Source: CAD feature listing. Evaluate the final solid. Frame: model axes, mm. A direction names the side the tool comes from. Give positions to 0.01 mm unless a question says otherwise; leave off trailing zeros. Order: outer loops, then holes, each group sorted by start corner. A loop starts at its lowest first (then second) coordinate and runs counter-clockwise, first axis right, second up.
from build123d import *

# Parameters (mm, degrees)
F0_R     = 15.875
F0_R_2   = 9.525
F1_DEPTH = 127
F2_R     = 9.525
F3_DEPTH = 12.7
F5_SCALE = 0.5


with BuildPart() as f1:
    # F0 (on Right) → F1 (new body)
    with BuildSketch(Plane.YZ):
        Circle(F0_R)
        Circle(F0_R_2, mode=Mode.SUBTRACT)
    extrude(amount=F1_DEPTH)

    # F2 (on face) → F3 (join)
    with BuildSketch(Plane.YZ.offset(127)):
        Polygon((-0.4526267682, -15.8685460584), (13.5162506236, -8.3262593089), (13.9688773918, 7.5422867496), (0.4526267682, 15.8685460584), (-13.5162506236, 8.3262593089), (-13.9688773918, -7.5422867496), align=None)
        Circle(F2_R, mode=Mode.SUBTRACT)
    extrude(amount=F3_DEPTH)

    # F4: F1 across face


with BuildPart() as f1_1:
    add(f1.part)
    add(f1.part.mirror(Plane.YZ.offset(139.7)))


with BuildPart() as f1_2:
    # F5: moved
    add(f1_1.part.scale(F5_SCALE))


solid = f1_2.part
(1) Section B-B, the plane x = 30. Return loops of the section in (y, z) (1 decimal), plus the area to 3 significant figures.
(2) Pin query (flat end, axial travel): pin 1 Ø3 at (x, z) = (62.5, 5) entering from -Y. Return the tip coordinate at first contact, or that it passes through.
(3) Line query: line 1 along Z through (x, y) = (35, 0); line 2 along Y through (x, z) = (109, -0.5); line 3 along Z through (x, y) = (77, -4). Output: solid intervals per line, ascending.
(4) Section C-C, the plane y = 1.5. Return loops of the section in (x, z).
(5) Access query for faces 4 (the flat face through (76.2, 4, 6)), 5 (the flat face through (63.5, -4, -6)), 6 (the flat face through (63.5, 4, -6)). Directions: +Z, -Z, +X, -X, +Y, -Y. A direction counts if a zero-diameter tool reaches every point of the face in a straight line with its end or side. Return the directions, or none.
(6) Draft query along X for faces 1 (the cylindrical face through (31.31, -1.72, -7.75)), 2 (the flat face through (69.939, -3.653, -5.824)), 3 (the flat face through (139.7, 0, -5)). Return one class per face: +X half, -X half, draft (parallel to the pull), parting line (faces both ways), or undercut.
(7) Section A-A, the plane z = 0. Return loops of the section in (x, y).
Checks:
1. outline: circle Ø15.9 at (0, 0); hole circle Ø9.5 at (0, 0)
1. area: 127 mm2
2. pin 1: stops at y = -7.12
3. line 1: z = -7.94 to -4.76, 4.76 to 7.94
3. line 2: y = -7.92 to -4.74, 4.74 to 7.92
3. line 3: z = -6.86 to -2.58, 2.58 to 6.86
4. outline: (0, -7.79) - (63.5, -7.79) - (63.5, -7) - (76.2, -7) - (76.2, -7.79) - (139.7, -7.79) - (139.7, -4.52) - (0, -4.52) - close; (0, 4.52) - (139.7, 4.52) - (139.7, 7.79) - (76.2, 7.79) - (76.2, 7.15) - (63.5, 7.15) - (63.5, 7.79) - (0, 7.79) - close
5. face 4: +Z, +Y
5. face 5: -Z, -Y
5. face 6: -Z, +Y
6. face 1: draft
6. face 2: undercut
6. face 3: +X half
7. outline: (0, -7.94) - (63.5, -7.94) - (63.5, -6.88) - (76.2, -6.88) - (76.2, -7.94) - (139.7, -7.94) - (139.7, -4.76) - (0, -4.76) - close; (0, 4.76) - (139.7, 4.76) - (139.7, 7.94) - (76.2, 7.94) - (76.2, 6.88) - (63.5, 6.88) - (63.5, 7.94) - (0, 7.94) - close
